from build123d import *

# Parameters (mm, degrees)
SKETCH2_R           = 16.8275
BOSS_EXTRUDE1_DEPTH = 7.874


with BuildPart() as part:
    # Sketch1 → Revolve1 (revolve)
    with BuildSketch(Plane.XY):
        Polygon((-46.228, -30.1625), (0, -30.1625), (0, -12.1539), (-17.78, -12.1539), (-17.78, -16.637), (-46.228, -16.8275), align=None)
    revolve(axis=Axis((-46.228, 0, 0), (1, 0, 0)))

    # Sketch2 → Boss-Extrude1 (add)
    with BuildSketch(Plane.ZY.offset(46.228)):
        Polygon((0, 34.09102474), (-24.105994772, 24.105994772), (-34.09102474, 0), (-24.105994772, -24.105994772), (0, -34.09102474), (24.105994772, -24.105994772), (34.09102474, 0), (24.105994772, 24.105994772), align=None)
        Circle(SKETCH2_R, mode=Mode.SUBTRACT)
    extrude(amount=-BOSS_EXTRUDE1_DEPTH)


solid = part.part
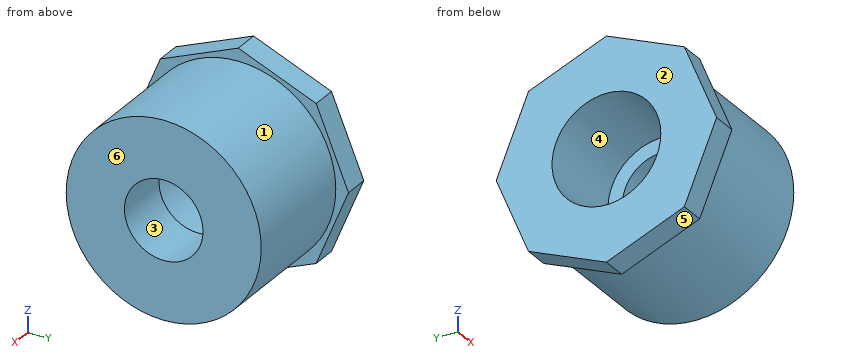
Design review of the part built by this model. Coordinates are the model's own, in mm. Face numbers are marked on the shaded views. A direction names the side the tool comes from. Round coordinates to 2 decimals unless told otherwise and drop trailing zeros. Loops run counter-clockwise (first coordinate to the right, second up) from the corner with the lowest first, then second, coordinate; pieces in that order, holes last. Notation, with made-up numbers: (-31.75, 75) - (9.25, 75) arc R18 cw to (9.25, 89) - close; hole circle Ø2 at (73.25, 64). An arc over 180 degrees is marked (long way). One line per item, written item: value. Start each with the question number.
1) Draft analysis for pull direction Y (two halves, no side actions). For the marked faces 3, 4, 5 and 6, state which applies: +Y half, -Y half, draft (parallel to the pull), parting line (faces both ways), or undercut.
2) Consider section C-C on y = -18.5. Give the boundary of the cut face in (x, z), then the cut area to 3 significant figures.
3) Insertion check: pin 1 Ø6 at (x, y) = (-28, 8.5) entering from -Z; pin 2 Ø2 at (x, z) = (-18, -19.5) entering from -Y; pin 3 Ø5 at (x, y) = (-19, 2.5) entering from +Z. Each pin has a flat end and moves straight along its axis. Give the tip position at first contact, or say it passes through.
4) Consider section A-A on x = -4.5. Give the boundary of the cut face in (y, z) (1 decimal), then the cut area to 3 significant figures.
5) Consider section B-B on y = 27.5. Give the boundary of the cut face in (x, z), then the cut area to 3 significant figures.
6) Consider section D-D on x = -25. Give the boundary of the cut face in (y, z) (1 decimal).
7) For the marked faces 1 and 2, list the 3-axis set-ups (+Z, -Z, +X, -X, +Y, -Y) from which the entire face can be reached by the end or side of a thin tool; tool diameter is ignored.
8) To check wall thickness, follow L1, parallel to Z at x = -8, y = 0; L2, parallel to X at y = -0.5, z = -12.5. State the ranges of each line that lie inside material, in increasing order. Write a range as from..to.
Reported:
1. face 3: undercut
1. face 4: undercut
1. face 5: -Y half
1. face 6: draft
2. outline: (-46.23, -26.43) - (-38.35, -26.43) - (-38.35, -23.82) - (0, -23.82) - (0, 23.82) - (-38.35, 23.82) - (-38.35, 26.43) - (-46.23, 26.43) - close
2. area: 2,240 mm^2
3. pin 1: stops at z = -29.66
3. pin 2: stops at y = -23.82
3. pin 3: stops at z = 30.16
4. outline: circle Ø60.3 at (0, 0); hole circle Ø24.3 at (0, 0)
4. area: 2,390 mm^2
5. outline: (-46.23, -15.91) - (-38.35, -15.91) - (-38.35, -12.39) - (0, -12.39) - (0, 12.39) - (-38.35, 12.39) - (-38.35, 15.91) - (-46.23, 15.91) - close
5. area: 1,200 mm^2
6. outline: circle Ø60.3 at (0, 0); hole circle Ø33.4 at (0, 0)
7. face 1: +X
7. face 2: +Z, -Z, -X, +Y, -Y
8. L1: z = -30.16..-12.15, 12.15..30.16
8. L2: x = -17.78..0
